```python
from build123d import *

# Parameters (mm, degrees)
F1_DEPTH = 1.5


with BuildPart() as f1:
    # F0 (on Front) → F1 (new body, symmetric)
    with BuildSketch(Plane.XZ):
        with BuildLine():
            Line((-118.194595, -20.131947), (-12.594595, -20.131947))
            Line((-12.594595, -20.131947), (-8.794595, -20.131947))
            Line((-8.794595, -20.131947), (-8.794595, 7.868053))
            Line((-8.794595, 7.868053), (-5.794595, 7.868053))
            Line((-5.794595, 7.868053), (-5.794595, -20.131947))
            Line((-5.794595, -20.131947), (103.605405, -20.131947))
            Line((103.605405, -20.131947), (103.605405, 7.868053))
            Line((103.605405, 7.868053), (106.605405, 7.868053))
            Line((106.605405, 7.868053), (106.605405, -20.131947))
            Line((106.605405, -20.131947), (216.005405, -20.131947))
            Line((216.005405, -20.131947), (216.005405, 7.868053))
            Line((216.005405, 7.868053), (219.005405, 7.868053))
            Line((219.005405, 7.868053), (219.005405, -20.131947))
            Line((219.005405, -20.131947), (328.405405, -20.131947))
            Line((328.405405, -20.131947), (336.602465, -10.363072))
            ThreePointArc((336.602465, -10.363072), (336.965365, -9.819955), (337.20211, -9.211166))
            Line((337.20211, -9.211166), (347.405405, 28.868053))
            Line((347.405405, 28.868053), (347.405405, 33.868053))
            ThreePointArc((347.405405, 33.868053), (346.819619, 35.282266), (345.405405, 35.868053))
            Line((345.405405, 35.868053), (-12.594595, 35.868053))
            Line((-12.594595, 35.868053), (-233.594595, 35.868053))
            Line((-233.594595, 35.868053), (-233.594595, 7.868053))
            Line((-233.594595, 7.868053), (-230.594595, 7.868053))
            Line((-230.594595, 7.868053), (-230.594595, -20.131947))
            Line((-230.594595, -20.131947), (-121.194595, -20.131947))
            Line((-121.194595, -20.131947), (-121.194595, 7.868053))
            Line((-121.194595, 7.868053), (-118.194595, 7.868053))
            Line((-118.194595, 7.868053), (-118.194595, -20.131947))
        make_face()
    extrude(amount=F1_DEPTH, both=True)


solid = f1.part
```
The model under review builds one solid part; all positions refer to its coordinate system, in mm. Give positions to 0.01 mm unless a question says otherwise; leave off trailing zeros. Write each loop counter-clockwise with the first axis right and the second up, starting at its lowest first coordinate (ties: lowest second). Pieces come first, ordered by that corner, then holes. Notation, with made-up numbers: (66, 45) - (109, 45) arc R28 ccw to (109, 79) - close; hole circle Ø1 at (-31.75, 86.25). An arc over 180 degrees is marked (long way). Answer in a Markdown table with one row per item. Add a question column.
1. Wall thickness on line 1 along X through (y, z) = (-0.8, -9); line 2 along X through (y, z) = (1.25, -1); line 3 along Z through (x, y) = (105, 0.7): over which ranges is each line inside the solid? List them lowest first. Write a range as [from, to].
2. We need section A-A on y = -0.2. Write out the cut boundary in (x, z), then the cut area to 3 significant figures.
3. Insertion check: P1, Ø1.5, axis at x = 105.5, y = -0.5, coming from the -Z side; P2, Ø1.5, axis at y = 0.5, z = -8.5, coming from the +X side; P3, Ø1.5, axis at y = 0.5, z = -1, coming from the -X side. Each pin has a flat end and moves straight along its axis. Give the tip position at first contact, or say it passes through.
Ans:
| question | item | result |
|---|---|---|
| 1 | line 1 | x = [-230.59, -121.19], [-118.19, -8.79], [-5.79, 103.61], [106.61, 216.01], [219.01, 337.26] |
| 1 | line 2 | x = [-230.59, -121.19], [-118.19, -8.79], [-5.79, 103.61], [106.61, 216.01], [219.01, 339.4] |
| 1 | line 3 | z = [7.87, 35.87] |
| 2 | outline | (-233.59, 7.87) - (-230.59, 7.87) - (-230.59, -20.13) - (-121.19, -20.13) - (-121.19, 7.87) - (-118.19, 7.87) - (-118.19, -20.13) - (-8.79, -20.13) - (-8.79, 7.87) - (-5.79, 7.87) - (-5.79, -20.13) - (103.61, -20.13) - (103.61, 7.87) - (106.61, 7.87) - (106.61, -20.13) - (216.01, -20.13) - (216.01, 7.87) - (219.01, 7.87) - (219.01, -20.13) - (328.41, -20.13) - (336.6, -10.36) arc R3 ccw to (337.2, -9.21) - (347.41, 28.87) - (347.41, 33.87) arc R2 ccw to (345.41, 35.87) - (-233.59, 35.87) - close |
| 2 | area | 31,800 mm^2 |
| 3 | P1 | stops at z = 7.87 |
| 3 | P2 | stops at x = 337.59 |
| 3 | P3 | stops at x = -230.59 |
